```python
from build123d import *

# Parameters (mm, degrees)
F0_W     = 70
F0_H     = 76
F0_R     = 2.25
F0_R_2   = 1.375
F0_R_3   = 0.875
F0_R_4   = 4
F0_R_5   = 6.5
F1_DEPTH = 13
F2_R     = 1.375
F2_R_2   = 0.875
F2_R_3   = 4
F2_W     = 50
F2_H     = 8.5
F3_DEPTH = 10
F4_R     = 3


with BuildPart() as f1:
    # F0 (on Top) → F1 (new body)
    with BuildSketch(Plane.XY):
        Rectangle(F0_W, F0_H)
        with Locations((-30, -32)):
            Circle(F0_R, mode=Mode.SUBTRACT)
        with Locations((30, -32)):
            Circle(F0_R, mode=Mode.SUBTRACT)
        with Locations((2.5, -17.5)):
            Circle(F0_R_2, mode=Mode.SUBTRACT)
        with Locations((18.5, -9)):
            Circle(F0_R_3, mode=Mode.SUBTRACT)
        with Locations((-12, 2)):
            Circle(F0_R_4, mode=Mode.SUBTRACT)
        with Locations((-23.325496177, 23.5334982232)):
            Circle(F0_R_2, mode=Mode.SUBTRACT)
        with Locations((-30, 32)):
            Circle(F0_R, mode=Mode.SUBTRACT)
        with Locations((-12, 27.5)):
            Circle(F0_R_5, mode=Mode.SUBTRACT)
        with Locations((-0.674503823, 31.4665017768)):
            Circle(F0_R_2, mode=Mode.SUBTRACT)
        with Locations((20, 6.25)):
            Circle(F0_R_3, mode=Mode.SUBTRACT)
        with Locations((0.9756591943, 23)):
            Circle(F0_R_3, mode=Mode.SUBTRACT)
        with Locations((14.25, 20.5)):
            Circle(F0_R_3, mode=Mode.SUBTRACT)
        with Locations((30, 32)):
            Circle(F0_R, mode=Mode.SUBTRACT)
    extrude(amount=F1_DEPTH)

    # F2 (on face) → F3 (cut)
    with BuildSketch(Plane.XY.offset(13)):
        with BuildLine():
            Line((-25, 27), (-32.5, 27))
            Line((-32.5, 27), (-32.5, -27))
            Line((-32.5, -27), (-25, -27))
            Line((-25, -27), (25, -27))
            Line((25, -27), (32.5, -27))
            Line((32.5, -27), (32.5, 27))
            Line((32.5, 27), (25, 27))
            Line((25, 27), (-5.5192593016, 27))
            ThreePointArc((-5.5192593016, 27), (-12, 21), (-18.4807406984, 27))
            Line((-18.4807406984, 27), (-25, 27))
        make_face()
        with Locations((2.5, -17.5)):
            Circle(F2_R, mode=Mode.SUBTRACT)
        with Locations((18.5, -9)):
            Circle(F2_R_2, mode=Mode.SUBTRACT)
        with Locations((-12, 2)):
            Circle(F2_R_3, mode=Mode.SUBTRACT)
        with Locations((-23.325496177, 23.5334982232)):
            Circle(F2_R, mode=Mode.SUBTRACT)
        with Locations((20, 6.25)):
            Circle(F2_R_2, mode=Mode.SUBTRACT)
        with Locations((0.9756591943, 23)):
            Circle(F2_R_2, mode=Mode.SUBTRACT)
        with Locations((14.25, 20.5)):
            Circle(F2_R_2, mode=Mode.SUBTRACT)
        with BuildLine():
            Line((-25, 35.5), (-25, 27))
            Line((-25, 27), (-18.4807406984, 27))
            ThreePointArc((-18.4807406984, 27), (-12.2501853916, 33.99518339), (-5.5, 27.5))
            ThreePointArc((-5.5, 27.5), (-5.50481661, 27.2498146084), (-5.5192593016, 27))
            Line((-5.5192593016, 27), (25, 27))
            Line((25, 27), (25, 35.5))
            Line((25, 35.5), (-25, 35.5))
        make_face()
        with Locations((-0.674503823, 31.4665017768)):
            Circle(F2_R, mode=Mode.SUBTRACT)
        with Locations((0, -31.25)):
            Rectangle(F2_W, F2_H)
    extrude(amount=-F3_DEPTH, mode=Mode.SUBTRACT)

    # F4
    f4_edges = [f1.edges().sort_by_distance(p)[0] for p in [
        (-25, 27, 8),
        (25, 27, 8),
        (-25, -27, 8),
        (25, -27, 8),
        (32.5, -27, 8),
        (32.5, 27, 8),
        (25, 35.5, 8),
        (-25, 35.5, 8),
        (-32.5, 27, 8),
        (-32.5, -27, 8),
        (-25, -35.5, 8),
        (25, -35.5, 8),
    ]]
    fillet(f4_edges, radius=F4_R)


solid = f1.part
```
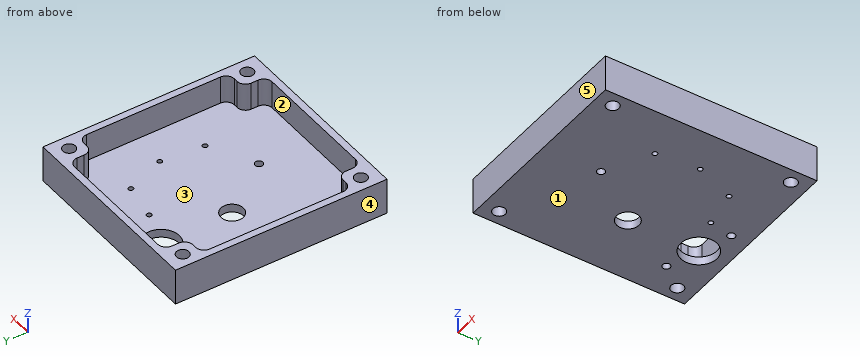
CAD build for the part. Positions are in the model's coordinates, mm. Face numbers are marked on the shaded views. A direction names the side the tool comes from. Coordinates: 2 decimals unless noted, no trailing zeros. Order: outer loops, then holes, each group sorted by start corner. A loop starts at its lowest first (then second) coordinate and runs counter-clockwise, first axis right, second up. Notation, with made-up numbers: (83, -38) - (98, -38) arc R8 cw to (98, -34) - close; hole circle Ø5 at (68, -5). An arc over 180 degrees is marked (long way). Use a Markdown table: item, result. Add a question column.
(1) Saw through at B-B (z = 10). Count the separate pieces of the cut face and the enclosed holes in it, then the cut area to 3 significant figures.
(2) Drill centre lines: line 1 along X through (y, z) = (-24, 4.25); line 2 along Y through (x, z) = (3.5, 8); line 3 along Y through (x, z) = (-30, 7.75). Where is each one in solid material? Low to high. Write a range as [from, to].
(3) Saw through at C-C (x = -23). Give the cut face in (y, z).
(4) Flat gauge pins, fed straight in: pin 1 (10.5 mm diameter, centred on x = -12, y = 27.5, fed in from -Z); pin 2 (3.5 mm diameter, centred on x = -0.67, y = 31.47, fed in from +Z). Where does each tip first touch, or does it go through?
(5) Saw through at D-D (y = 17). Give the cut face in (x, z), then the cut area to 3 significant figures.
(6) Saw through at A-A (y = -9). Give the cut face in (x, z) (3 decimals).
(7) Pull direction X, two halves, no side cores. Call the marked faces 3, 4 and 5: +X half, -X half, draft (parallel to the pull), parting line (faces both ways), or undercut.
(8) Which spindle directions (+Z, -Z, +X, -X, +Y, -Y) get a long thin tool onto all of the face, cutting with end or side? Do the marked faces 1 and 2. Say none if no direction does.
Solved:
| question | item | result |
|---|---|---|
| 1 | separate pieces | 1 |
| 1 | enclosed holes | 5 |
| 1 | area | 904 mm² |
| 2 | line 1 | x = [-35, -32.5], [32.5, 35] |
| 2 | line 2 | y = [-38, -35.5], [35.5, 38] |
| 2 | line 3 | y = [-38, -34.25], [-29.75, -26.96], [26.96, 29.75], [34.25, 38] |
| 3 | outline | (-38, 0) - (22.2, 0) - (22.2, 3) - (-35.33, 3) - (-35.33, 13) - (-38, 13) - close; (24.87, 0) - (38, 0) - (38, 13) - (35.33, 13) - (35.33, 3) - (24.87, 3) - close |
| 4 | pin 1 | passes through |
| 4 | pin 2 | stops at z = 3 |
| 5 | outline | (-35, 0) - (35, 0) - (35, 13) - (32.5, 13) - (32.5, 3) - (-32.5, 3) - (-32.5, 13) - (-35, 13) - close |
| 5 | area | 260 mm² |
| 6 | outline | (-35, 0) - (17.625, 0) - (17.625, 3) - (-32.5, 3) - (-32.5, 13) - (-35, 13) - close; (19.375, 0) - (35, 0) - (35, 13) - (32.5, 13) - (32.5, 3) - (19.375, 3) - close |
| 7 | face 3 | undercut |
| 7 | face 4 | -X half |
| 7 | face 5 | draft |
| 8 | face 1 | -Z, +X, -X, +Y, -Y |
| 8 | face 2 | +Z |
